For this review, take the finished solid that the model builds, in its own axes (mm). Face numbers are marked on the shaded views. A direction names the side the tool comes from. Give positions to 0.01 mm unless a question says otherwise; leave off trailing zeros. Loops run counter-clockwise (first coordinate to the right, second up) from the corner with the lowest first, then second, coordinate; pieces in that order, holes last. Notation, with made-up numbers: (-24.5, 14) - (-15.5, 14) arc R16 ccw to (-15.5, 26) - close; hole circle Ø9 at (63, 35.25). An arc over 180 degrees is marked (long way). Use CSV: the item, a comma, the result in double quotes. Start each with the question number.
1. Mouldability with a two-part tool opening along Y and no side actions: class the marked faces 3, 4 and 5 as pulls with the +Y half, pulls with the -Y half, needs draft (parallel to the pull), parting line crosses it, or undercut.
2. Take a section at C-C on y = 17. Give the boundary of the cut face in (x, z) (3 decimals), plus the area to 3 significant figures.
3. Take a section at A-A on x = -56. Give the boundary of the cut face in (y, z) (1 decimal), plus the area to 3 significant figures.
4. Wall thickness on line 1 (Y direction, x = 35, z = 23.5); line 2 (X direction, y = -29.5, z = 19); line 3 (Z direction, x = -5, y = -10.5) (3 decimals): over which ranges is each line inside the solid? List them lowest first.
5. For pin 1 (6 mm diameter, centred on x = 50.5, y = -12, fed in from +Z) (3 decimals), flat-tipped, find the tip position at first contact; note if it passes through.
6. For the marked faces 1 and 2, list the 3-axis set-ups (+Z, -Z, +X, -X, +Y, -Y) from which the entire face can be reached by the end or side of a thin tool; tool diameter is ignored.
7. Take a section at B-B on z = 13.75. Give the boundary of the cut face in (x, y).
8. Take a section at D-D on y = -5.5. Give the boundary of the cut face in (x, z) (3 decimals), plus the area to 3 significant figures.
```python
from build123d import *

# Parameters (mm, degrees)
F1_DEPTH = 3.175
F2_DEPTH = 25.4


with BuildPart() as f1:
    # F0 (on Top) → F1 (new body)
    with BuildSketch(Plane.XY):
        Polygon((62.195573, -39.6875), (62.195573, 39.6875), (-67.979427, 39.6875), (-67.979427, 14.3002), (-67.979427, 0), (-67.979427, -14.3002), (-67.979427, -39.6875), (-2.891927, -39.6875), align=None)
        Polygon((-67.979427, 0), (-67.979427, 14.3002), (-71.154427, 14.3002), (-71.154427, -14.3002), (-67.979427, -14.3002), align=None)
    extrude(amount=F1_DEPTH)

    # F0 (on Top) → F2 (join)
    with BuildSketch(Plane.XY):
        Polygon((-67.979427, 39.6875), (62.195573, 39.6875), (62.195573, -39.6875), (-2.891927, -39.6875), (-67.979427, -39.6875), (-67.979427, -14.3002), (-71.154427, -14.3002), (-71.154427, -42.8625), (65.370573, -42.8625), (65.370573, 42.8625), (-71.154427, 42.8625), (-71.154427, 14.3002), (-67.979427, 14.3002), align=None)
    extrude(amount=F2_DEPTH)


solid = f1.part
```
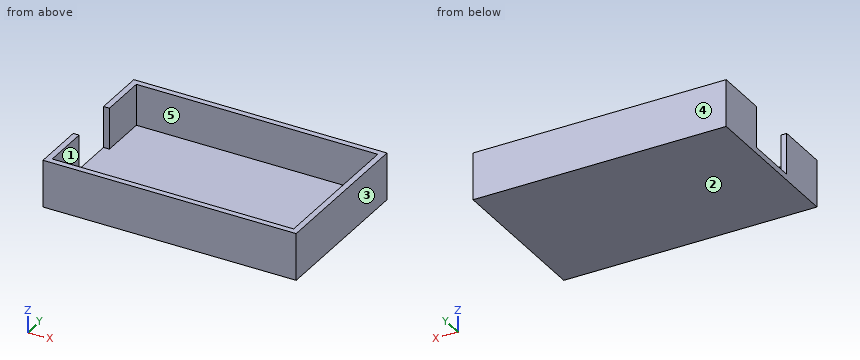
Check result:
1,face 3,"needs draft"
1,face 4,"pulls with the +Y half"
1,face 5,"undercut"
2,outline,"(-71.154, 0) - (65.371, 0) - (65.371, 25.4) - (62.196, 25.4) - (62.196, 3.175) - (-67.979, 3.175) - (-67.979, 25.4) - (-71.154, 25.4) - close"
2,area,"575 mm²"
3,outline,"(-42.9, 0) - (42.9, 0) - (42.9, 25.4) - (39.7, 25.4) - (39.7, 3.2) - (-39.7, 3.2) - (-39.7, 25.4) - (-42.9, 25.4) - close"
3,area,"413 mm²"
4,line 1,"y = -42.86 to -39.69, 39.69 to 42.86"
4,line 2,"x = -71.15 to -67.98, 62.2 to 65.37"
4,line 3,"z = 0 to 3.175"
5,pin 1,"stops at z = 3.175"
6,face 1,"+Z"
6,face 2,"-Z, +X, -X, +Y, -Y"
7,outline,"(-71.15, -42.86) - (65.37, -42.86) - (65.37, 42.86) - (-71.15, 42.86) - (-71.15, 14.3) - (-67.98, 14.3) - (-67.98, 39.69) - (62.2, 39.69) - (62.2, -39.69) - (-67.98, -39.69) - (-67.98, -14.3) - (-71.15, -14.3) - close"
8,outline,"(-71.154, 0) - (65.371, 0) - (65.371, 25.4) - (62.196, 25.4) - (62.196, 3.175) - (-71.154, 3.175) - close"
8,area,"504 mm²"
